Geometry check sheet. Reference: the model listing, model coordinates, mm. Give positions to 0.01 mm unless a question says otherwise; leave off trailing zeros. Loops run counter-clockwise (first coordinate to the right, second up) from the corner with the lowest first, then second, coordinate; pieces in that order, holes last. Notation, with made-up numbers: (-39, -20.75) -> (-22, -20.75) arc R23 ccw to (-22, 16.25) -> close; hole circle Ø2 at (34.25, -2). An arc over 180 degrees is marked (long way). One line per item, written item: value. Start each with the question number.
(1) Sectioned sample at C-C, the plane x = 42.5. Record the cut outline in (y, z).
(2) Gauge pin test, flat ends, axial feed: pin 1 Ø1.6 at (x, z) = (32.5, -5.5) entering from +Y; pin 2 Ø0.6 at (x, y) = (-8, -1) entering from -Z; pin 3 Ø1 at (y, z) = (-1, -1) entering from +X; pin 4 Ø0.6 at (y, z) = (-1, 2) entering from -X. Record the tip position at first contact, or that the pin passes through.
(3) Sectioned sample at D-D, the plane x = 25. Record the cut outline in (y, z).
(4) Sectioned sample at B-B, the plane z = 7.75. Record the cut outline in (x, y).
(5) Sectioned sample at A-A, the plane y = -1.3. State how many separate pieces and enclosed holes the cut face has, then the cut area to 3 significant figures.
(6) Scan lines: line 1 along X through (y, z) = (-1.35, 3.75); line 2 along Z through (x, y) = (25, -0.9); line 3 along X through (y, z) = (-0.4, -7). Record each from-to range of solid material in increasing order. Write a range as from..to.
from build123d import *

# Parameters (mm, degrees)
F0_R     = 1
F0_R_2   = 1.5
F1_DEPTH = 2


with BuildPart() as f1:
    # F0 (on Front) → F1 (new body)
    with BuildSketch(Plane.XZ):
        with BuildLine():
            ThreePointArc((-21, 10), (-20.853553, 10.353553), (-20.5, 10.5))
            Line((-20.5, 10.5), (20.5, 10.5))
            ThreePointArc((20.5, 10.5), (20.853553, 10.353553), (21, 10))
            Line((21, 10), (21, -10))
            ThreePointArc((21, -10), (21.146447, -10.353553), (21.5, -10.5))
            Line((21.5, -10.5), (30, -10.5))
            Line((30, -10.5), (45, -10.5))
            Line((45, -10.5), (48, -10.5))
            Line((48, -10.5), (48, -2.894959))
            ThreePointArc((48, -2.894959), (47.327048, -0.389634), (45.489338, 1.441306))
            Line((45.489338, 1.441306), (22.156183, 14.836265))
            ThreePointArc((22.156183, 14.836265), (20.954997, 15.331218), (19.666845, 15.5))
            Line((19.666845, 15.5), (0, 15.5))
            Line((0, 15.5), (-19.666845, 15.5))
            ThreePointArc((-19.666845, 15.5), (-20.954997, 15.331218), (-22.156183, 14.836265))
            Line((-22.156183, 14.836265), (-45.489338, 1.441306))
            ThreePointArc((-45.489338, 1.441306), (-47.327048, -0.389634), (-48, -2.894959))
            Line((-48, -2.894959), (-48, -10.5))
            Line((-48, -10.5), (-45, -10.5))
            Line((-45, -10.5), (-30, -10.5))
            Line((-30, -10.5), (-21.5, -10.5))
            ThreePointArc((-21.5, -10.5), (-21.146447, -10.353553), (-21, -10))
            Line((-21, -10), (-21, 10))
        make_face()
        with Locations((-42.5, -5.5)):
            Circle(F0_R, mode=Mode.SUBTRACT)
        with Locations((-32.5, -5.5)):
            Circle(F0_R, mode=Mode.SUBTRACT)
        with Locations((-25, -5)):
            Circle(F0_R_2, mode=Mode.SUBTRACT)
        with Locations((25, -5)):
            Circle(F0_R_2, mode=Mode.SUBTRACT)
        with Locations((32.5, -5.5)):
            Circle(F0_R, mode=Mode.SUBTRACT)
        with Locations((42.5, -5.5)):
            Circle(F0_R, mode=Mode.SUBTRACT)
        with Locations((-25, 5)):
            Circle(F0_R_2, mode=Mode.SUBTRACT)
        with Locations((25, 5)):
            Circle(F0_R_2, mode=Mode.SUBTRACT)
    extrude(amount=F1_DEPTH)


solid = f1.part
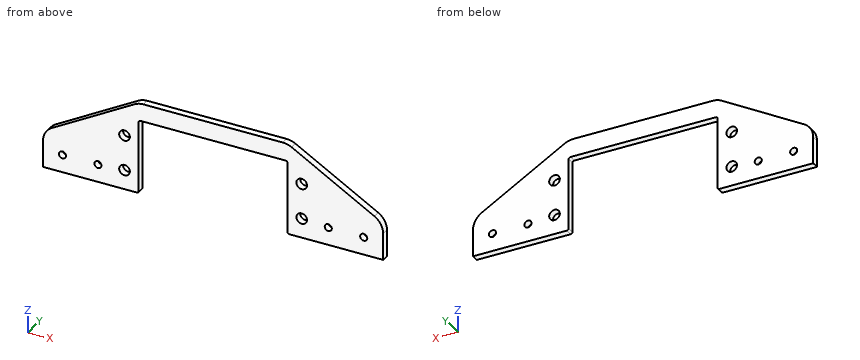
Calculated:
1. outline: (-2, -10.5) -> (0, -10.5) -> (0, -6.5) -> (-2, -6.5) -> close; (-2, -4.5) -> (0, -4.5) -> (0, 3.16) -> (-2, 3.16) -> close
2. pin 1: passes through
2. pin 2: stops at z = 10.5
2. pin 3: stops at x = 47.8
2. pin 4: stops at x = -45.04
3. outline: (-2, -10.5) -> (0, -10.5) -> (0, -6.5) -> (-2, -6.5) -> close; (-2, -3.5) -> (0, -3.5) -> (0, 3.5) -> (-2, 3.5) -> close; (-2, 6.5) -> (0, 6.5) -> (0, 13.2) -> (-2, 13.2) -> close
4. outline: (-34.5, -2) -> (-21, -2) -> (-21, 0) -> (-34.5, 0) -> close; (21, -2) -> (34.5, -2) -> (34.5, 0) -> (21, 0) -> close
5. separate pieces: 1
5. enclosed holes: 8
5. area: 1,150 mm2
6. line 1: x = -41.47..-25.83, -24.17..-21, 21..24.17, 25.83..41.47
6. line 2: z = -10.5..-6.5, -3.5..3.5, 6.5..13.2
6. line 3: x = -48..-21, 21..48
